Autodesk Inventor part; units mm, degrees
ref_plane "YZ Plane" through (0, 0, 0) normal (1, 0, 0) x (0, 1, 0)
ref_plane "XZ Plane" through (0, 0, 0) normal (0, 1, 0) x (-1, 0, 0)
ref_plane "XY Plane" through (0, 0, 0) normal (0, 0, 1) x (1, 0, 0)
sketch "Sketch1" plane through (0, 0, 0) normal (1, 0, 0) x (0, 1, 0)
  circle A0 centre (0, 0) radius 76.2
  line L0 (0, 0) -> (44.7892, 61.6471) construction
  line L1 (0, 0) -> (-44.7892, 61.6471) construction
  line L2 (0, 0) -> (-26.0619, 71.6046) construction
  line L3 (0, -76.2) -> (0, 76.2) construction
  line L4 (-10.5331, 28.9395) -> (-17.4277, 47.8823)
  arc A1 (13.9724, 54.4354) -> (-13.9724, 54.4354) centre (0, 0) ccw
  arc A2 (4.8996, 25.7378) -> (-4.8996, 25.7378) centre (0, 0) ccw
  arc A3 (17.4277, 47.8823) -> (13.9724, 54.4354) centre (12.7293, 49.5924) ccw
  arc A4 (4.8996, 25.7378) -> (10.5331, 28.9395) centre (5.8346, 30.6496) ccw
  arc A5 (-10.5331, 28.9395) -> (-4.8996, 25.7378) centre (-5.8346, 30.6496) ccw
  arc A6 (-13.9724, 54.4354) -> (-17.4277, 47.8823) centre (-12.7293, 49.5924) ccw
  line L5 (0, 0) -> (26.0619, 71.6046) construction
  line L6 (17.4277, 47.8823) -> (10.5331, 28.9395)
  line L7 (-32.7534, 39.034) -> (-19.7958, 23.5917)
  arc A7 (-32.7534, 39.034) -> (-40.1563, 39.3181) centre (-36.5836, 35.8201) ccw
  arc A8 (-19.8398, 17.1121) -> (-19.7958, 23.5917) centre (-23.626, 20.3777) ccw
  line L8 (-30.3289, 5.3478) -> (-50.1811, 8.8483)
  arc A9 (-30.3289, 5.3478) -> (-24.7394, 8.6257) centre (-29.4606, 10.2718) ccw
  arc A10 (-19.8398, 17.1121) -> (-24.7394, 8.6257) centre (0, 0) ccw
  arc A11 (-40.1563, 39.3181) -> (-54.1286, 15.1173) centre (0, 0) ccw
  arc A12 (-54.1286, 15.1173) -> (-50.1811, 8.8483) centre (-49.3129, 13.7723) ccw
  line L9 (-50.1811, -8.8483) -> (-30.3289, -5.3478)
  arc A13 (-50.1811, -8.8483) -> (-54.1286, -15.1173) centre (-49.3129, -13.7723) ccw
  arc A14 (-24.7394, -8.6257) -> (-30.3289, -5.3478) centre (-29.4606, -10.2718) ccw
  line L10 (-19.7958, -23.5917) -> (-32.7534, -39.034)
  arc A15 (-19.7958, -23.5917) -> (-19.8398, -17.1121) centre (-23.626, -20.3777) ccw
  arc A16 (-24.7394, -8.6257) -> (-19.8398, -17.1121) centre (0, 0) ccw
  arc A17 (-54.1286, -15.1173) -> (-40.1563, -39.3181) centre (0, 0) ccw
  arc A18 (-40.1563, -39.3181) -> (-32.7534, -39.034) centre (-36.5836, -35.8201) ccw
  line L11 (-17.4277, -47.8823) -> (-10.5331, -28.9395)
  arc A19 (-17.4277, -47.8823) -> (-13.9724, -54.4354) centre (-12.7293, -49.5924) ccw
  arc A20 (-4.8996, -25.7378) -> (-10.5331, -28.9395) centre (-5.8346, -30.6496) ccw
  line L12 (10.5331, -28.9395) -> (17.4277, -47.8823)
  arc A21 (10.5331, -28.9395) -> (4.8996, -25.7378) centre (5.8346, -30.6496) ccw
  arc A22 (-4.8996, -25.7378) -> (4.8996, -25.7378) centre (0, 0) ccw
  arc A23 (-13.9724, -54.4354) -> (13.9724, -54.4354) centre (0, 0) ccw
  arc A24 (13.9724, -54.4354) -> (17.4277, -47.8823) centre (12.7293, -49.5924) ccw
  line L13 (32.7534, -39.034) -> (19.7958, -23.5917)
  arc A25 (32.7534, -39.034) -> (40.1563, -39.3181) centre (36.5836, -35.8201) ccw
  arc A26 (19.8398, -17.1121) -> (19.7958, -23.5917) centre (23.626, -20.3777) ccw
  line L14 (30.3289, -5.3478) -> (50.1811, -8.8483)
  arc A27 (30.3289, -5.3478) -> (24.7394, -8.6257) centre (29.4606, -10.2718) ccw
  arc A28 (19.8398, -17.1121) -> (24.7394, -8.6257) centre (0, 0) ccw
  arc A29 (40.1563, -39.3181) -> (54.1286, -15.1173) centre (0, 0) ccw
  arc A30 (54.1286, -15.1173) -> (50.1811, -8.8483) centre (49.3129, -13.7723) ccw
  circle A31 centre (0, 0) radius 10
  circle A32 centre (0, 0) radius 26.2 construction
  line L15 (50.1811, 8.8483) -> (30.3289, 5.3478)
  arc A33 (50.1811, 8.8483) -> (54.1286, 15.1173) centre (49.3129, 13.7723) ccw
  arc A34 (24.7394, 8.6257) -> (30.3289, 5.3478) centre (29.4606, 10.2718) ccw
  line L16 (19.7958, 23.5917) -> (32.7534, 39.034)
  arc A35 (19.7958, 23.5917) -> (19.8398, 17.1121) centre (23.626, 20.3777) ccw
  arc A36 (24.7394, 8.6257) -> (19.8398, 17.1121) centre (0, 0) ccw
  arc A37 (54.1286, 15.1173) -> (40.1563, 39.3181) centre (0, 0) ccw
  arc A38 (40.1563, 39.3181) -> (32.7534, 39.034) centre (36.5836, 35.8201) ccw
  point P0 (8.9609, 24.6199)
  point P1 (-8.9609, 24.6199)
  point P2 (-19.2215, 52.8107)
  dimension "d1" = 72
  dimension "d4" = 16
  dimension "d7" = 20
  dimension "d8" = 152.4
  dimension "d9" = 30
  dimension "d10" = 5
  dimension "d11" = 5
  dimension "d12" = 36
  dimension "d13" = 20
  dimension "d16" = 360
  dimension "d18" = 20
  dimension "d21" = 52.4
extrude "Extrusion2" add sketch "Sketch1" along normal blind 6.35
properties part number "paddlewheel_outer"
For this review, take the finished solid that the model builds, in its own axes (mm). Round coordinates to 2 decimals unless told otherwise and drop trailing zeros. Write each loop counter-clockwise with the first axis right and the second up, starting at its lowest first coordinate (ties: lowest second). Pieces come first, ordered by that corner, then holes. Notation, with made-up numbers: M 59.5,22.25 L 110.5,22.25 A12 ccw 110.5,39.25 Z; hole C 33.5,76 d8. An arc over 180 degrees is marked long. One line per item, written item: value. Start each with the question number.
(1) We need section C-C (x = 2). Count the separate pieces of the cut face and the enclosed holes in it, and give its area (3 significant figures).
(2) Wall thickness on line 1 (Z direction, x = 4, y = 0); line 2 (Y direction, x = 4.5, z = 19); line 3 (Y direction, x = 2.75, z = -34): over which ranges is each line inside the solid? List them lowest first.
(3) We need section D-D (z = 66.5). Give the boundary of the cut face in (x, y).
(4) We need section A-A (y = 0). Give the boundary of the cut face in (x, z), and give its area (3 significant figures).
(5) We need section B-B (z = 0). Give the boundary of the cut face in (x, y), and give its area (3 significant figures).
(6) The part is to be moulded in two halves that separate along Z. For faces 1 (the flat face through (0, -1, -16)), 2 (the cylindrical face through (3.131, -26.889, 5.984)), say which applies: released by +Z, released by -Z, zero draft, split by the parting line, or undercut.
(7) Insertion check: pin 1 (3 mm diameter, centred on x = 0.5, y = -13, fed in from -Z); pin 2 (8 mm diameter, centred on y = -39, z = -44, fed in from -X); pin 3 (1.5 mm diameter, centred on x = 4, y = -35, fed in from +Z); pin 4 (12 mm diameter, centred on y = 0, z = 0, fed in from -X). Each pin has a flat end and moves straight along its axis. Give the tip position at first contact, or say it passes through.
Result:
1. separate pieces: 1
1. enclosed holes: 7
1. area: 12,900 mm²
2. line 1: -76.2 to -56.2, -26.2 to -10, 10 to 26.2, 56.2 to 76.2
2. line 2: -73.79 to -52.89, -18.82 to 18.82, 52.89 to 73.79
2. line 3: -68.19 to -44.75, -28.53 to -12.37, 12.37 to 28.53, 44.75 to 68.19
3. outline: M 0,-37.2 L 6.35,-37.2 L 6.35,37.2 L 0,37.2 Z
4. outline: M 0,-76.2 L 6.35,-76.2 L 6.35,-56.2 L 0,-56.2 Z; M 0,-26.2 L 6.35,-26.2 L 6.35,-10 L 0,-10 Z; M 0,10 L 6.35,10 L 6.35,26.2 L 0,26.2 Z; M 0,56.2 L 6.35,56.2 L 6.35,76.2 L 0,76.2 Z
4. area: 460 mm²
5. outline: M 0,-76.2 L 6.35,-76.2 L 6.35,-10 L 0,-10 Z; M 0,10 L 6.35,10 L 6.35,76.2 L 0,76.2 Z
5. area: 841 mm²
6. face 1: zero draft
6. face 2: undercut
7. pin 1: z = -75.33
7. pin 2: x = 0
7. pin 3: z = 68.07
7. pin 4: through
